Read the model definition and answer for the solid it produces. Units are mm, in the model's axes. A direction names the side the tool comes from. Coordinates: 2 decimals unless noted, no trailing zeros. Write each loop counter-clockwise with the first axis right and the second up, starting at its lowest first coordinate (ties: lowest second). Pieces come first, ordered by that corner, then holes. Notation, with made-up numbers: (36.25, 8) -> (41.25, 8) arc R15 cw to (41.25, 19) -> close; hole circle Ø9 at (-40, -3.5). An arc over 180 degrees is marked (long way). Return JSON: item names as keys, results as strings.
from build123d import *

# Parameters (mm, degrees)
SKETCH21_R           = 1.7
SKETCH21_W           = 27.57
SKETCH21_H           = 9.66
BOSS_EXTRUDE18_DEPTH = 6


with BuildPart() as part:
    # Sketch21 → Boss-Extrude18 (new body)
    with BuildSketch(Plane(origin=(0, 0, 0), x_dir=(1, 0, 0), z_dir=(0, 1, 0))):
        Polygon((-16.06, -12.06), (-16.06, 20.06), (-16.06, 84), (0, 84), (16.06, 84), (16.06, 20.06), (80, 20.06), (80, 4), (80, -12.06), (16.06, -12.06), (16.06, -76), (0, -76), (-16.06, -76), align=None)
        with Locations(Location((-12.56, 36.04, 0), (0, 0, 270))):
            Circle(SKETCH21_R, mode=Mode.SUBTRACT)
        with Locations(Location((12.56, 36.04, 0), (0, 0, 270))):
            Circle(SKETCH21_R, mode=Mode.SUBTRACT)
        with Locations(Location((12.56, -12.97, 0), (0, 0, 270))):
            Circle(SKETCH21_R, mode=Mode.SUBTRACT)
        with Locations(Location((-12.56, -12.97, 0), (0, 0, 270))):
            Circle(SKETCH21_R, mode=Mode.SUBTRACT)
        with Locations((0, 25.47)):
            Rectangle(SKETCH21_W, SKETCH21_H, mode=Mode.SUBTRACT)
    extrude(amount=BOSS_EXTRUDE18_DEPTH)


solid = part.part
1. The part is cut by section B-B (z = -36.04). Determine the outline of the cut face in (x, y), then the cut area to 3 significant figures.
Taken from the geometry:
{"outline": "(-16.06, 0) -> (-14.26, 0) -> (-14.26, 6) -> (-16.06, 6) -> close; (-10.86, 0) -> (10.86, 0) -> (10.86, 6) -> (-10.86, 6) -> close; (14.26, 0) -> (16.06, 0) -> (16.06, 6) -> (14.26, 6) -> close", "area": "152 mm2"}
2. Flat-ended cylindrical pins translate along their axes: pin 1 Ø1.8 at (x, y) = (40, 3.5) entering from -Z; pin 2 Ø5.5 at (x, z) = (12.56, 12.97) entering from -Y; pin 3 Ø1 at (x, y) = (42, 4.5) entering from +Z; pin 4 Ø1.8 at (y, z) = (3.5, 35.5) entering from +X. Find the tip coordinate at first contact, or state that the pin passes through.
Taken from the geometry:
{"pin 1": "stops at z = -20.06", "pin 2": "stops at y = 0", "pin 3": "stops at z = 12.06", "pin 4": "stops at x = 16.06"}
3. The part is cut by section C-C (y = 4.1). Determine the outline of the cut face in (x, z) (3 decimals).
Taken from the geometry:
{"outline": "(-16.06, -84) -> (16.06, -84) -> (16.06, -20.06) -> (80, -20.06) -> (80, 12.06) -> (16.06, 12.06) -> (16.06, 76) -> (-16.06, 76) -> close; hole circle Ø3.4 at (-12.56, -36.04); hole circle Ø3.4 at (-12.56, 12.97); hole (-13.785, -30.3) -> (13.785, -30.3) -> (13.785, -20.64) -> (-13.785, -20.64) -> close; hole circle Ø3.4 at (12.56, -36.04); hole circle Ø3.4 at (12.56, 12.97)"}
4. Consider L1, parallel to X at y = 1.7, z = 12.97; L2, parallel to Z at x = -6, y = 3.9; L3, parallel to X at y = 0.9, z = 40. Determine where each line is inside the solid, lowest interval first.
Taken from the geometry:
{"L1": "x = -16.06 to -14.26, -10.86 to 10.86, 14.26 to 16.06", "L2": "z = -84 to -30.3, -20.64 to 76", "L3": "x = -16.06 to 16.06"}
5. The part is cut by section D-D (x = 36.5). Determine the outline of the cut face in (y, z).
Taken from the geometry:
{"outline": "(0, -20.06) -> (6, -20.06) -> (6, 12.06) -> (0, 12.06) -> close"}
6. A tool of negligible diameter and unlimited length cuts with its end or side. For faces 4 (the face through (16.06, 3, -52)), 5 (the face through (48, 3, 12.06)), 6 (the face through (0, 3, -20.64)), from which of +Z, -Z, +X, -X, +Y, -Y can it reach the whole face along a straight path? Write none if from no direction.
Taken from the geometry:
{"face 4": "-Z, +X, +Y, -Y", "face 5": "+Z, +X, +Y, -Y", "face 6": "+Y, -Y"}
7. The part is cut by section A-A (x = 5). Determine the outline of the cut face in (y, z).
Taken from the geometry:
{"outline": "(0, -84) -> (6, -84) -> (6, -30.3) -> (0, -30.3) -> close; (0, -20.64) -> (6, -20.64) -> (6, 76) -> (0, 76) -> close"}
8. For a pull along X with two mould halves and no side action, classify faces 1 (the face through (80, 3, -4)), 2 (the face through (-12.49, 2.96, 11.27)), 3 (the face through (48, 3, -20.06)) as +X half, -X half, draft (parallel to the pull), parting line (faces both ways), or undercut.
Taken from the geometry:
{"face 1": "+X half", "face 2": "undercut", "face 3": "draft"}
